from build123d import *

# Parameters (mm, degrees)
EXTRUDE_THIN1_DEPTH = 90
CUT_EXTRUDE1_DEPTH  = 180.484492174
SKETCH3_R           = 2
SKETCH3_W           = 35
SKETCH3_H           = 14
SKETCH3_W_2         = 38
SKETCH3_H_2         = 50
CUT_EXTRUDE2_DEPTH  = 135.593407947
BOSS_EXTRUDE1_REACH = 156.207
SKETCH4_R           = 3


with BuildPart() as part:
    # Sketch1 → Extrude-Thin1 (new body)
    with BuildSketch(Plane.XY):
        with BuildLine():
            Line((-67.681421148, -71.208727913), (-67.681421148, -10))
            ThreePointArc((-67.681421148, -10), (-64.75248896, -2.928932188), (-57.681421148, 0))
            Line((-57.681421148, 0), (60.318578852, 0))
            ThreePointArc((60.318578852, 0), (67.389646664, -2.928932188), (70.318578852, -10))
            Line((70.318578852, -10), (70.318578852, -68))
            Line((70.318578852, -68), (67.318578852, -68))
            Line((67.318578852, -68), (67.318578852, -10))
            ThreePointArc((67.318578852, -10), (65.268326321, -5.050252532), (60.318578852, -3))
            Line((60.318578852, -3), (-57.681421148, -3))
            ThreePointArc((-57.681421148, -3), (-62.631168616, -5.050252532), (-64.681421148, -10))
            Line((-64.681421148, -10), (-64.681421148, -71.208727913))
            Line((-64.681421148, -71.208727913), (-67.681421148, -71.208727913))
        make_face()
    extrude(amount=EXTRUDE_THIN1_DEPTH)

    # Sketch2 → Cut-Extrude1 (cut, through all)
    with BuildSketch(Plane.ZY.offset(67.681421148)):
        Polygon((90, -71.208727913), (90, -10), (27.119645112, -57.791474126), (19.564108931, -47.850479311), (13.348687597, -64.736940064), (7.43570584, -62.560541261), (1.525048388, -70.700264204), (0, -71.469431607), align=None)
    extrude(amount=-CUT_EXTRUDE1_DEPTH, mode=Mode.SUBTRACT)

    # Sketch3 → Cut-Extrude2 (cut, through all)
    with BuildSketch(Plane(origin=(0, 0, 0), x_dir=(1, 0, 0), z_dir=(0, 1, 0))):
        with Locations(Location((26, -20, 0), (0, 0, 180))):
            Circle(SKETCH3_R)
        with Locations(Location((-26, -20, 0), (0, 0, 180))):
            Circle(SKETCH3_R)
        with Locations((52.818578852, -83)):
            Rectangle(SKETCH3_W, SKETCH3_H)
        with Locations((-50.181421148, -83)):
            Rectangle(SKETCH3_W, SKETCH3_H)
        with Locations((0, -65)):
            Rectangle(SKETCH3_W_2, SKETCH3_H_2)
    extrude(amount=-CUT_EXTRUDE2_DEPTH, mode=Mode.SUBTRACT)

    # Boss-Extrude1: up to this face of the body (flat: up to its plane)
    boss_extrude1_end = Plane(part.part.faces().sort_by_distance((35.318578852, -1.5, 83))[0])
    # Sketch4 → Boss-Extrude1 (add, up to the picked face)
    with BuildSketch(Plane.ZY.offset(32.681421148), mode=Mode.PRIVATE) as boss_extrude1_sk1:
        with Locations(Location((90, -1.5, 0), (0, 0, 150))):
            Circle(SKETCH4_R)
    boss_extrude1_tool1 = split(extrude(boss_extrude1_sk1.sketch, amount=-BOSS_EXTRUDE1_REACH, mode=Mode.PRIVATE), bisect_by=boss_extrude1_end, keep=Keep.BOTH, mode=Mode.PRIVATE)
    add(boss_extrude1_tool1.solids().sort_by(Axis((-32.681421, -1.5, 90), (1, 0, 0)))[0])


solid = part.part
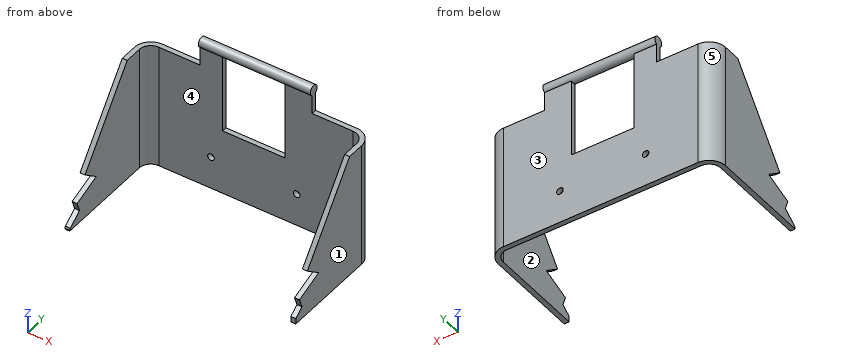
Part model, mm, in its own coordinate system. Face numbers are marked on the shaded views. A direction names the side the tool comes from. Coordinates: 2 decimals unless noted, no trailing zeros. Write each loop counter-clockwise with the first axis right and the second up, starting at its lowest first coordinate (ties: lowest second). Pieces come first, ordered by that corner, then holes. Notation, with made-up numbers: M 47.5,-25.75 L 63.5,-25.75 A21 cw 63.5,-3.75 Z; hole C -5,75 d5. An arc over 180 degrees is marked long. Return JSON: item names as keys, results as strings.
1. 3-axis set-ups, long thin cutter, end or side, ignore diameter. For the marked faces 1 and 2: which of +Z, -Z, +X, -X, +Y, -Y reach the whole face in a straight line?
Determined:
{"face 1": "+Z, -Z, +X, +Y, -Y", "face 2": "+Z, -Z, -Y"}
2. Probe L1, parallel to X at y = -33, z = 49; L2, parallel to Z at x = 26, y = -1.7; L3, parallel to Y at x = -53, z = 50. List the from-to ranges inside material, lowest first.
Determined:
{"L1": "-67.68 to -64.68, 67.32 to 70.32", "L2": "0 to 18, 22 to 92.99", "L3": "-3 to 0"}
3. Saw through at D-D, the plane y = -49.5. Write the cut outline in (x, z), then the cut area to 3 significant figures.
Determined:
{"outline": "M -67.68,0 L -64.68,0 L -64.68,18.96 L -67.68,18.96 Z; M -67.68,20.82 L -64.68,20.82 L -64.68,38.03 L -67.68,38.03 Z; M 67.32,0 L 70.32,0 L 70.32,18.96 L 67.32,18.96 Z; M 67.32,20.82 L 70.32,20.82 L 70.32,38.03 L 67.32,38.03 Z", "area": "217 mm²"}
4. Saw through at B-B, the plane y = -15.5. Write the cut outline in (x, z).
Determined:
{"outline": "M -67.68,0 L -64.68,0 L -64.68,76 L -67.68,76 Z; M 67.32,0 L 70.32,0 L 70.32,76 L 67.32,76 Z"}
5. Flat gauge pins, fed straight in: pin 1 Ø10 at (x, z) = (37, 42.5) entering from -Y; pin 2 Ø10.5 at (x, y) = (61, -7) entering from +Z; pin 3 Ø5 at (y, z) = (-2.5, 87.5) entering from +X. Where does each tip first touch, or does it go through?
Determined:
{"pin 1": "y = -3", "pin 2": "z = 76", "pin 3": "x = 35.32"}
6. Saw through at A-A, the plane x = 3. Write the cut outline in (y, z).
Determined:
{"outline": "C -1.5,90 d6; M -3,0 L 0,0 L 0,40 L -3,40 Z"}
7. Saw through at C-C, the plane z = 44.5. Write the cut outline in (x, y).
Determined:
{"outline": "M -67.68,-44.58 L -64.68,-44.58 L -64.68,-10 A7 cw -57.68,-3 L -19,-3 L -19,0 L -57.68,0 A10 ccw -67.68,-10 Z; M 19,-3 L 60.32,-3 A7 cw 67.32,-10 L 67.32,-44.58 L 70.32,-44.58 L 70.32,-10 A10 ccw 60.32,0 L 19,0 Z"}
8. Pull direction X, two halves, no side cores. Call the marked faces 3, 4 and 5: pulls with the +X half, pulls with the -X half, needs draft (parallel to the pull), parting line crosses it, or undercut.
Determined:
{"face 3": "needs draft", "face 4": "undercut", "face 5": "pulls with the -X half"}
